from build123d import *

# Parameters (mm, degrees)
SKETCH1_W           = 113
SKETCH1_H           = 204
BOSS_EXTRUDE1_DEPTH = 3
SKETCH2_W           = 10
SKETCH2_H           = 3
BOSS_EXTRUDE2_DEPTH = 3
LPATTERN1_COUNT     = 10
LPATTERN1_PITCH     = 20
SKETCH4_W           = 103
SKETCH4_H           = 20
CUT_EXTRUDE1_DEPTH  = 4
SKETCH3_W           = 12
SKETCH3_H           = 3
SKETCH3_W_2         = 10
BOSS_EXTRUDE3_DEPTH = 3


with BuildPart() as part:
    # Sketch1 → Boss-Extrude1 (new body)
    with BuildSketch(Plane(origin=(0, 0, 0), x_dir=(1, 0, 0), z_dir=(0, 1, 0))):
        with Locations((56.5, 102)):
            Rectangle(SKETCH1_W, SKETCH1_H)
    extrude(amount=BOSS_EXTRUDE1_DEPTH)

    # Sketch2 → Boss-Extrude2 (add)
    with BuildSketch(Plane(origin=(113, 0, 0), x_dir=(0, 0, -1), z_dir=(1, 0, 0))):
        with Locations((12, 1.5)):
            Rectangle(SKETCH2_W, SKETCH2_H)
    boss_extrude2 = extrude(amount=BOSS_EXTRUDE2_DEPTH)

    # LPattern1: Boss-Extrude2 ×10
    with Locations(*[(0, 0, -i * LPATTERN1_PITCH) for i in range(1, LPATTERN1_COUNT)]):
        add(boss_extrude2)

    # Sketch4 → Cut-Extrude1 (cut, through all)
    with BuildSketch(Plane(origin=(0, 3, 0), x_dir=(1, 0, 0), z_dir=(0, 1, 0))):
        with Locations((56.5, 15)):
            Rectangle(SKETCH4_W, SKETCH4_H)
        with Locations((56.5, 189)):
            Rectangle(SKETCH4_W, SKETCH4_H)
    extrude(amount=-CUT_EXTRUDE1_DEPTH, mode=Mode.SUBTRACT)

    # Sketch3 → Boss-Extrude3 (add)
    with BuildSketch(Plane.ZY):
        with Locations((-6, 1.5)):
            Rectangle(SKETCH3_W, SKETCH3_H)
        with Locations((-27, 1.5)):
            Rectangle(SKETCH3_W_2, SKETCH3_H)
        with Locations((-47, 1.5)):
            Rectangle(SKETCH3_W_2, SKETCH3_H)
        with Locations((-67, 1.5)):
            Rectangle(SKETCH3_W_2, SKETCH3_H)
        with Locations((-87, 1.5)):
            Rectangle(SKETCH3_W_2, SKETCH3_H)
        with Locations((-107, 1.5)):
            Rectangle(SKETCH3_W_2, SKETCH3_H)
        with Locations((-127, 1.5)):
            Rectangle(SKETCH3_W_2, SKETCH3_H)
        with Locations((-147, 1.5)):
            Rectangle(SKETCH3_W_2, SKETCH3_H)
        with Locations((-167, 1.5)):
            Rectangle(SKETCH3_W_2, SKETCH3_H)
        with Locations((-187, 1.5)):
            Rectangle(SKETCH3_W_2, SKETCH3_H)
    extrude(amount=BOSS_EXTRUDE3_DEPTH)


solid = part.part
Read the model definition and answer for the solid it produces. Units are mm, in the model's axes. Give positions to 0.01 mm unless a question says otherwise; leave off trailing zeros. Write each loop counter-clockwise with the first axis right and the second up, starting at its lowest first coordinate (ties: lowest second). Pieces come first, ordered by that corner, then holes. Notation, with made-up numbers: (-1.5, 77) -> (50.5, 77) arc R22 ccw to (50.5, 110) -> close; hole circle Ø4 at (12, 55.5). An arc over 180 degrees is marked (long way). Answer as a JSON object with one key per item and string values. Group by question number.
1) Each of these flat-tipped pins is pushed along its axis until it touches: P1, Ø0.9, axis at x = 114, y = 2, coming from the -Z side; P2, Ø1.5, axis at x = -1.5, y = 2, coming from the +Z side; P3, Ø0.9, axis at y = 1.5, z = -35.5, coming from the -X side; P4, Ø1.5, axis at y = 1.5, z = -123, coming from the +X side. Where does it stop, or does it pass through?
2) Consider L1, parallel to Z at x = 6, y = 0.55; L2, parallel to X at y = 1.15, z = -157.5; L3, parallel to X at y = 1.1, z = -35. Determine where each line is inside the solid, lowest interval first. Write a range as from..to.
3) Find section A-A (x = 61.5). Write down the section's boundary in (y, z).
4) Find section B-B (z = -35). Write down the section's boundary in (x, y).
5) Find section C-C (y = 0.75). Count the separate pieces of the cut face and the enclosed holes in it, and give its area (3 significant figures).
Values follow:
{
 "1": {"P1": "stops at z = -197", "P2": "stops at z = 0", "P3": "stops at x = 0", "P4": "stops at x = 113"},
 "2": {"L1": "z = -204..-199, -179..-25, -5..0", "L2": "x = 0..113", "L3": "x = 0..116"},
 "3": {"outline": "(0, -204) -> (3, -204) -> (3, -199) -> (0, -199) -> close; (0, -179) -> (3, -179) -> (3, -25) -> (0, -25) -> close; (0, -5) -> (3, -5) -> (3, 0) -> (0, 0) -> close"},
 "4": {"outline": "(0, 0) -> (116, 0) -> (116, 3) -> (0, 3) -> close"},
 "5": {"separate pieces": "1", "enclosed holes": "2", "area": "19,500 mm2"}
}
